from build123d import *

# Parameters (mm, degrees)
SKETCH1_W           = 424
SKETCH1_H           = 295
SKETCH1_W_2         = 61
SKETCH1_H_2         = 142
BOSS_EXTRUDE1_DEPTH = 10


with BuildPart() as part:
    # Sketch1 → Boss-Extrude1 (new body)
    with BuildSketch(Plane(origin=(0, 0, 0), x_dir=(1, 0, 0), z_dir=(0, 1, 0))):
        Rectangle(SKETCH1_W, SKETCH1_H)
        with Locations((-151.5, 73.5)):
            Rectangle(SKETCH1_W_2, SKETCH1_H_2, mode=Mode.SUBTRACT)
        with Locations((-75.75, 73.5)):
            Rectangle(SKETCH1_W_2, SKETCH1_H_2, mode=Mode.SUBTRACT)
        with Locations((0, 73.5)):
            Rectangle(SKETCH1_W_2, SKETCH1_H_2, mode=Mode.SUBTRACT)
        with Locations((75.75, 73.5)):
            Rectangle(SKETCH1_W_2, SKETCH1_H_2, mode=Mode.SUBTRACT)
        with Locations((151.5, 73.5)):
            Rectangle(SKETCH1_W_2, SKETCH1_H_2, mode=Mode.SUBTRACT)
        with Locations((151.5, -73.5)):
            Rectangle(SKETCH1_W_2, SKETCH1_H_2, mode=Mode.SUBTRACT)
        with Locations((75.75, -73.5)):
            Rectangle(SKETCH1_W_2, SKETCH1_H_2, mode=Mode.SUBTRACT)
        with Locations((0, -73.5)):
            Rectangle(SKETCH1_W_2, SKETCH1_H_2, mode=Mode.SUBTRACT)
        with Locations((-75.75, -73.5)):
            Rectangle(SKETCH1_W_2, SKETCH1_H_2, mode=Mode.SUBTRACT)
        with Locations((-151.5, -73.5)):
            Rectangle(SKETCH1_W_2, SKETCH1_H_2, mode=Mode.SUBTRACT)
    extrude(amount=BOSS_EXTRUDE1_DEPTH)


solid = part.part
Design review of the part built by this model. Coordinates are the model's own, in mm. A direction names the side the tool comes from. Give positions to 0.01 mm unless a question says otherwise; leave off trailing zeros. Order: outer loops, then holes, each group sorted by start corner. A loop starts at its lowest first (then second) coordinate and runs counter-clockwise, first axis right, second up.
1. To check wall thickness, follow L1, parallel to X at y = 9, z = 44.5; L2, parallel to Z at x = 90, y = 8. State the ranges of each line that lie inside material, in increasing order.
Solution:
L1: x = -212 to -182, -121 to -106.25, -45.25 to -30.5, 30.5 to 45.25, 106.25 to 121, 182 to 212
L2: z = -147.5 to -144.5, -2.5 to 2.5, 144.5 to 147.5
2. Mouldability with a two-part tool opening along Z and no side actions: class faces 3 (the flat face through (-3, 0, -2)), 4 (the flat face through (-30.5, 5, -73)), 5 (the flat face through (0, 5, -2.5)) as +Z half, -Z half, draft (parallel to the pull), parting line (faces both ways), or undercut.
Solution:
face 3: draft
face 4: undercut
face 5: undercut
3. Add section C-C, the plane y = 5. State how many separate pieces and enclosed holes the cut face has, then the cut area to 3 significant figures.
Solution:
separate pieces: 1
enclosed holes: 10
area: 38,500 mm2
4. Add section B-B, the plane x = -51. State the section outline as (y, z) points, then the cut area to 3 significant figures.
Solution:
outline: (0, -147.5) - (10, -147.5) - (10, -144.5) - (0, -144.5) - close; (0, -2.5) - (10, -2.5) - (10, 2.5) - (0, 2.5) - close; (0, 144.5) - (10, 144.5) - (10, 147.5) - (0, 147.5) - close
area: 110 mm2
5. Add section A-A, the plane z = 83.5. State the section outline as (x, y) points.
Solution:
outline: (-212, 0) - (-182, 0) - (-182, 10) - (-212, 10) - close; (-121, 0) - (-106.25, 0) - (-106.25, 10) - (-121, 10) - close; (-45.25, 0) - (-30.5, 0) - (-30.5, 10) - (-45.25, 10) - close; (30.5, 0) - (45.25, 0) - (45.25, 10) - (30.5, 10) - close; (106.25, 0) - (121, 0) - (121, 10) - (106.25, 10) - close; (182, 0) - (212, 0) - (212, 10) - (182, 10) - close
6. Tool access review of faces 1 (the flat face through (-212, 5, 2)), 2 (the flat face through (75, 5, -144.5)): name each direction out of +Z, -Z, +X, -X, +Y, -Y from which nothing blocks a thin tool from reaching the whole face with its end or side.
Solution:
face 1: +Z, -Z, -X, +Y, -Y
face 2: +Y, -Y
